from build123d import *

# Parameters (mm, degrees)
CYLINDER001_R     = 2.2
CYLINDER001_DEPTH = 5
CYLINDER002_R     = 1.175
CYLINDER002_DEPTH = 5
BOX004_W          = 5.5
BOX004_H          = 5
BOX004_DEPTH      = 3.5
CYLINDER_R        = 2.9
CYLINDER_DEPTH    = 4
BOX003_W          = 13
BOX003_H          = 14
BOX003_DEPTH      = 7
BOX002_W          = 13
BOX002_H          = 14
BOX002_DEPTH      = 10
BOX001_W          = 13
BOX001_H          = 40
BOX001_DEPTH      = 1.75
BOX_W             = 13
BOX_H             = 28
BOX_DEPTH         = 20
CYLINDER003_W     = 3.875
CYLINDER003_H     = 3
CYLINDER003_ANGLE = 180


with BuildPart() as taladro_master:
    # Cylinder001 → Cylinder001 (new body)
    with BuildSketch(Plane(origin=(0, -17.35, 18), x_dir=(1, 0, 0), z_dir=(0, 0, 1))):
        Circle(CYLINDER001_R)
    extrude(amount=CYLINDER001_DEPTH)


with BuildPart() as obj1:
    # Cylinder002 → Cylinder002 (new body)
    with BuildSketch(Plane(origin=(0, 7, 29.5), x_dir=(1, 0, 0), z_dir=(0, 0, 1))):
        Circle(CYLINDER002_R)
    extrude(amount=CYLINDER002_DEPTH)


with BuildPart() as fusion_huecos:
    # Part__Mirroring: instance of Taladro master
    add(taladro_master.part.mirror(Plane(origin=(0, 0, 0), x_dir=(1, 0, 0), z_dir=(0, 1, 0))))

    # Fusion001: union Taladro master, obj1
    add(taladro_master.part)
    add(obj1.part)


with BuildPart() as obj2:
    # Box004 → Box004 (new body)
    with BuildSketch(Plane(origin=(3.75, 28, 4), x_dir=(1, 0, 0), z_dir=(0, 0, 1))):
        with Locations((2.75, 2.5)):
            Rectangle(BOX004_W, BOX004_H)
    extrude(amount=BOX004_DEPTH)


with BuildPart() as cilindro:
    # Cylinder → Cylinder (new body)
    with BuildSketch(Plane(origin=(6.5, 21, 30), x_dir=(1, 0, 0), z_dir=(0, 0, 1))):
        Circle(CYLINDER_R)
    extrude(amount=CYLINDER_DEPTH)


with BuildPart() as obj3:
    # Box003 → Box003 (new body)
    with BuildSketch(Plane.XY.offset(20)):
        with Locations((6.5, 7)):
            Rectangle(BOX003_W, BOX003_H)
    extrude(amount=BOX003_DEPTH)


with BuildPart() as cubo_eje:
    # Box002 → Box002 (new body)
    with BuildSketch(Plane(origin=(0, 14, 20), x_dir=(1, 0, 0), z_dir=(0, 0, 1))):
        with Locations((6.5, 7)):
            Rectangle(BOX002_W, BOX002_H)
    extrude(amount=BOX002_DEPTH)


with BuildPart() as obj4:
    # Box001 → Box001 (new body)
    with BuildSketch(Plane(origin=(0, -6, 20), x_dir=(1, 0, 0), z_dir=(0, 0, 1))):
        with Locations((6.5, 20)):
            Rectangle(BOX001_W, BOX001_H)
    extrude(amount=BOX001_DEPTH)


with BuildPart() as obj5:
    # Box → Box (new body)
    with BuildSketch(Plane.XY):
        with Locations((6.5, 14)):
            Rectangle(BOX_W, BOX_H)
    extrude(amount=BOX_DEPTH)


with BuildPart() as servo_hd1160a_master:
    # Cylinder003 → Cylinder003 (revolve)
    with BuildSketch(Plane(origin=(6.5, 14, 27), x_dir=(-1, 0, 0), z_dir=(0, 1, 0))):
        with Locations((1.9375, 1.5)):
            Rectangle(CYLINDER003_W, CYLINDER003_H)
    revolve(axis=Axis((6.5, 14, 27), (0, 0, 1)), revolution_arc=CYLINDER003_ANGLE)

    # Fusion: union obj2, Cilindro, obj3, Cubo eje, obj4, obj5
    add(obj2.part)
    add(cilindro.part)
    add(obj3.part)
    add(cubo_eje.part)
    add(obj4.part)
    add(obj5.part)


with BuildPart() as servo_hd1160a_master_1:
    # Fusion placement: moved
    add(servo_hd1160a_master.part.moved(Location((-6.5, -14, 0))))

    # Cut: cut Fusion huecos
    add(fusion_huecos.part, mode=Mode.SUBTRACT)


with BuildPart() as servo_hd1160a_master_2:
    # Cut placement: moved
    add(servo_hd1160a_master_1.part.moved(Location((0, -7, 0))))


solid = servo_hd1160a_master_2.part
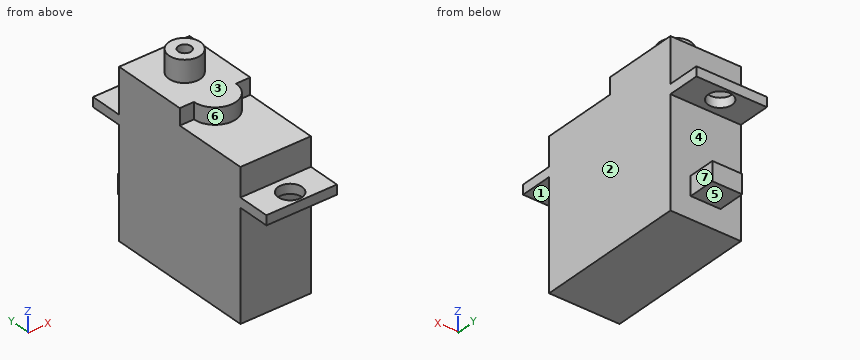
Can you work these out from the model? Positions are in its coordinate system, mm. Face numbers are marked on the shaded views. A direction names the side the tool comes from. Coordinates: 2 decimals unless noted, no trailing zeros. Loops run counter-clockwise (first coordinate to the right, second up) from the corner with the lowest first, then second, coordinate; pieces in that order, holes last. Notation, with made-up numbers: M 12,22.25 L 58,22.25 A27 ccw 58,50.25 Z; hole C 77,-9.75 d6. An arc over 180 degrees is marked long. Answer as CSV lines item,"result". Start each with the question number.
1. Suppose I cut it at C-C, the plane x = 5. List the corners of the cut face in (y, z) for me, plus the area to 3 significant figures.
2. Suppose I cut it at D-D, the plane y = 0. List the corners of the cut face in (x, z) for me (3 decimals).
3. If I drill on probe 1 along Y at (x, z) = (0, 20.75); probe 2 along X at (y, z) = (-24.35, 20.9); probe 3 along Y at (x, z) = (0, 31.55) (3 decimals), over which ranges is the centre line in solid material (lowest first)? Write a range as [from, to].
4. For the marked faces 5, 6 and 7, which set-ups out of +Z, -Z, +X, -X, +Y, -Y let a thin tool reach every point of the face, with its end or its side?
5. Thinking about a two-plate mould opening in Z: for the marked faces 1, 2, 3 and 4, which applies, +Z half, -Z half, draft (parallel to the pull), parting line (faces both ways), or undercut?
6. For pin 1 Ø4 at (x, y) = (0, 10) entering from -Z; pin 2 Ø3 at (x, z) = (5.5, 29) entering from -Y; pin 3 Ø4 at (x, z) = (-3, 27.5) entering from +Y; pin 4 Ø6.5 at (x, y) = (2.5, 9) entering from -Z, each with a flat end and sliding along its axis, tell me the tip position at first contact or that it passes through.
7. Suppose I cut it at B-B, the plane y = -24.35. List the corners of the cut face in (x, z) for me.
8. Suppose I cut it at A-A, the plane y = 10.35. List the corners of the cut face in (x, z) for me, plus the area to 3 significant figures.
Output:
1,outline,"M -27,20 L -21,20 L -21,0 L 7,0 L 7,20 L 13,20 L 13,21.75 L 7,21.75 L 7,30 L -7,30 L -7,27 L -21,27 L -21,21.75 L -27,21.75 Z"
1,area,"819 mm^2"
2,outline,"M -6.5,0 L 6.5,0 L 6.5,30 L 2.9,30 L 2.9,34 L 1.175,34 L 1.175,29.5 L -1.175,29.5 L -1.175,34 L -2.9,34 L -2.9,30 L -6.5,30 Z"
3,probe 1,"y = [-27, -26.55], [-22.15, 8.15], [12.55, 13]"
3,probe 2,"x = [-6.5, -2.2], [2.2, 6.5]"
3,probe 3,"y = [-2.9, -1.175], [1.175, 2.9]"
4,face 5,"-Z, +X, -X, +Y"
4,face 6,"+Z, -Y"
4,face 7,"-Z, +X, +Y"
5,face 1,"-Z half"
5,face 2,"draft"
5,face 3,"+Z half"
5,face 4,"undercut"
6,pin 1,"stops at z = 4"
6,pin 2,"stops at y = -7"
6,pin 3,"stops at y = 7"
6,pin 4,"stops at z = 0"
7,outline,"M -6.5,20 L -2.2,20 L -2.2,21.75 L -6.5,21.75 Z; M 2.2,20 L 6.5,20 L 6.5,21.75 L 2.2,21.75 Z"
8,outline,"M -6.5,20 L -2.2,20 L -2.2,21.75 L -6.5,21.75 Z; M -2.75,4 L 2.75,4 L 2.75,7.5 L -2.75,7.5 Z; M 2.2,20 L 6.5,20 L 6.5,21.75 L 2.2,21.75 Z"
8,area,"34.3 mm^2"
